```python
from build123d import *

# Parameters (mm, degrees)
SKETCH1_W           = 38.1
SKETCH1_H           = 88.9
BOSS_EXTRUDE1_DEPTH = 1143
SKETCH2_R           = 21.43125
CUT_EXTRUDE4_DEPTH  = 1145.498323502
FILLET1_R           = 3.175


with BuildPart() as part:
    # Sketch1 → Boss-Extrude1 (new body)
    with BuildSketch(Plane(origin=(0, 0, 0), x_dir=(1, 0, 0), z_dir=(0, 1, 0))):
        Rectangle(SKETCH1_W, SKETCH1_H)
    extrude(amount=BOSS_EXTRUDE1_DEPTH)

    # Sketch2 → Cut-Extrude4 (cut, through all)
    with BuildSketch(Plane(origin=(-19.05, 0, 0), x_dir=(0, 0, -1), z_dir=(1, 0, 0))):
        with Locations(Location((12.7, 458.7875, 0), (0, 0, 180))):
            Circle(SKETCH2_R)
        with Locations(Location((12.7, 939.8, 0), (0, 0, 180))):
            Circle(SKETCH2_R)
    extrude(amount=CUT_EXTRUDE4_DEPTH, mode=Mode.SUBTRACT)

    # Fillet1
    fillet1_edges = [part.edges().sort_by_distance(p)[0] for p in [
        (19.05, 571.5, 44.45),
        (-19.05, 571.5, 44.45),
        (-19.05, 571.5, -44.45),
        (19.05, 571.5, -44.45),
    ]]
    fillet(fillet1_edges, radius=FILLET1_R)


solid = part.part
```
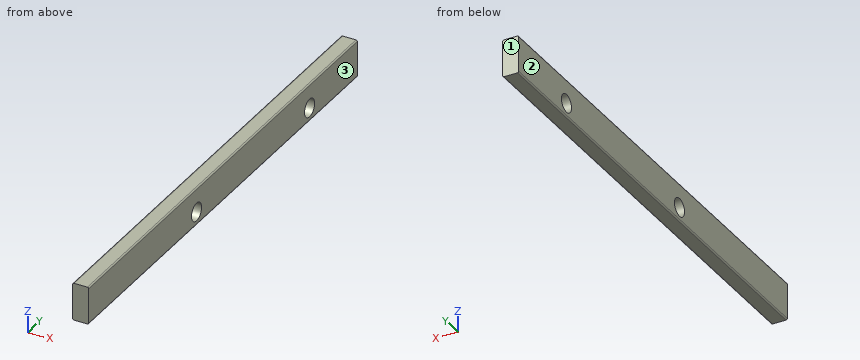
Design review of the part built by this model. Coordinates are the model's own, in mm. Face numbers are marked on the shaded views. Round coordinates to 2 decimals unless told otherwise and drop trailing zeros. Write each loop counter-clockwise with the first axis right and the second up, starting at its lowest first coordinate (ties: lowest second). Pieces come first, ordered by that corner, then holes.
Item 1: We need section C-C on x = 1.5. Write out the cut boundary in (y, z).
Item 2: We need section B-B on z = -12.7. Write out the cut boundary in (x, y).
Item 3: For probe 1 along Y at (x, z) = (5, -12); probe 2 along Z at (x, y) = (-5, 939.8); probe 3 along Z at (x, y) = (-15.5, 937), list the stretches that pass through material, from the lowest coordinate up.
Item 4: The part is to be moulded in two halves that separate along X. For the marked faces 1, 2 and 3, say which applies: +X half, -X half, draft (parallel to the pull), parting line (faces both ways), or undercut.
Item 5: We need section A-A on y = 939.8. Write out the cut boundary in (x, z) (3 decimals), and give its area (3 significant figures).
Returned:
1. outline: (0, -44.45) - (1143, -44.45) - (1143, 44.45) - (0, 44.45) - close; hole circle Ø42.86 at (458.79, -12.7); hole circle Ø42.86 at (939.8, -12.7)
2. outline: (-19.05, 0) - (19.05, 0) - (19.05, 437.36) - (-19.05, 437.36) - close; (-19.05, 480.22) - (19.05, 480.22) - (19.05, 918.37) - (-19.05, 918.37) - close; (-19.05, 961.23) - (19.05, 961.23) - (19.05, 1143) - (-19.05, 1143) - close
3. probe 1: y = 0 to 437.37, 480.21 to 918.38, 961.22 to 1143
3. probe 2: z = -44.45 to -34.13, 8.73 to 44.45
3. probe 3: z = -44.45 to -33.95, 8.55 to 44.45
4. face 1: draft
4. face 2: -X half
4. face 3: +X half
5. outline: (-19.05, -41.275) arc R3.175 ccw to (-15.875, -44.45) - (15.875, -44.45) arc R3.175 ccw to (19.05, -41.275) - (19.05, -34.131) - (-19.05, -34.131) - close; (-19.05, 8.731) - (19.05, 8.731) - (19.05, 41.275) arc R3.175 ccw to (15.875, 44.45) - (-15.875, 44.45) arc R3.175 ccw to (-19.05, 41.275) - close
5. area: 1,750 mm2
